Autodesk Inventor part; units mm, degrees
ref_plane "YZ Plane" through (0, 0, 0) normal (1, 0, 0) x (0, 1, 0)
ref_plane "XZ Plane" through (0, 0, 0) normal (0, 1, 0) x (-1, 0, 0)
ref_plane "XY Plane" through (0, 0, 0) normal (0, 0, 1) x (1, 0, 0)
sketch "Sketch1" plane through (0, 0, 0) normal (0, 0, 1) x (1, 0, 0)
  line L0 (-63.5, -76.2) -> (63.5, -76.2)
  line L1 (63.5, -76.2) -> (63.5, 76.2)
  line L2 (63.5, 76.2) -> (-63.5, 76.2)
  line L3 (-63.5, 76.2) -> (-63.5, -76.2)
  line L4 (-63.5, -76.2) -> (63.5, 76.2) construction
  line L5 (63.5, -76.2) -> (-63.5, 76.2) construction
  line L6 (-63.5, 76.2) -> (-50.0296, 62.7296)
  line L7 (-63.5, 76.2) -> (-44.45, 76.2) construction
  line L8 (63.5, 76.2) -> (69.85, 76.2) construction
  line L9 (63.5, 76.2) -> (50.0296, 62.7296)
  line L10 (63.5, -76.2) -> (50.0296, -62.7296)
  line L11 (-63.5, -76.2) -> (-50.0296, -62.7296)
  circle A0 centre (-50.0296, 62.7296) radius 3.175
  circle A1 centre (50.0296, 62.7296) radius 3.175
  circle A2 centre (50.0296, -62.7296) radius 3.175
  circle A3 centre (-50.0296, -62.7296) radius 3.175
  circle A4 centre (0, 0) radius 12.7
  line L12 (0, 0) -> (-48.4, 0) construction
  line L13 (0, 0) -> (12.7, 0)
  line L14 (0, 0) -> (49, 0) construction
  line L15 (49, 0) -> (49, 28.29) construction
  line L16 (49, 0) -> (49, -28.29) construction
  circle A5 centre (49, -28.29) radius 2.4
  circle A6 centre (49, 28.29) radius 2.4
  circle A7 centre (-48.4, 0) radius 2.4
  dimension "d10" = 25.4
  dimension "d0" = 127
  dimension "d1" = 152.4
  dimension "d2" = 19.05
  dimension "d3" = 45
  dimension "d6" = 6.35
  dimension "d7" = 6.35
  dimension "d8" = 6.35
  dimension "d9" = 6.35
  dimension "d11" = 48.4
  dimension "d12" = 49
  dimension "d13" = 28.29
  dimension "d14" = 28.29
  dimension "d15" = 4.8
  dimension "d16" = 4.8
  dimension "d17" = 4.8
extrude "Extrusion1" add sketch "Sketch1" along normal blind 6.35
properties part number "small plate"
Geometry check sheet. Reference: the model listing, model coordinates, mm. Coordinates: 2 decimals unless noted, no trailing zeros. Loops run counter-clockwise (first coordinate to the right, second up) from the corner with the lowest first, then second, coordinate; pieces in that order, holes last. Notation, with made-up numbers: (68.25, -8) - (109.25, -8) arc R29 ccw to (109.25, 23) - close; hole circle Ø11 at (80, 11.25). An arc over 180 degrees is marked (long way). One line per item, written item: value. Start each with the question number.
(1) Mould release check, pull along Y, two halves, no side actions. Record for faces 1 (the cylindrical face through (-50.798, -0.106, 3.131)), 2 (the flat face through (-63.5, 1, 3)), 3 (the flat face through (1, 76.2, 3)): released by +Y, released by -Y, zero draft, split by the parting line, or undercut.
(2) Depth check by flat-ended pin: P1, Ø8.5, axis at x = 50.03, y = 62.73, coming from the +Z side; P2, Ø23, axis at x = 0, y = 0, coming from the -Z side. Enter the tip coordinate at first touch or a pass-through.
(3) Cross-section at B-B on x = 0. Enter the section's corners in (y, z), plus the area to 3 significant figures.
(4) Material ranges on line 1 (X direction, y = -60, z = 5); line 2 (Y direction, x = 52.5, z = 2.25); line 3 (Y direction, x = 49, z = 4.5), recorded low to high. Write a range as [from, to].
(5) Cross-section at A-A on y = -28.29. Enter the section's corners in (x, z), plus the area to 3 significant figures.
(6) Cross-section at D-D on x = 49. Enter the section's corners in (y, z).
(7) Cross-section at C-C on z = 3. Count the separate pieces of the cut face and the enclosed holes in it, plus the area to 3 significant figures.
Results below:
1. face 1: undercut
1. face 2: zero draft
1. face 3: released by +Y
2. P1: stops at z = 6.35
2. P2: passes through
3. outline: (-76.2, 0) - (-12.7, 0) - (-12.7, 6.35) - (-76.2, 6.35) - close; (12.7, 0) - (76.2, 0) - (76.2, 6.35) - (12.7, 6.35) - close
3. area: 806 mm2
4. line 1: x = [-63.5, -51.65], [-48.41, 48.41], [51.65, 63.5]
4. line 2: y = [-76.2, -64.72], [-60.74, 60.74], [64.72, 76.2]
4. line 3: y = [-76.2, -65.73], [-59.73, -30.69], [-25.89, 25.89], [30.69, 59.73], [65.73, 76.2]
5. outline: (-63.5, 0) - (46.6, 0) - (46.6, 6.35) - (-63.5, 6.35) - close; (51.4, 0) - (63.5, 0) - (63.5, 6.35) - (51.4, 6.35) - close
5. area: 776 mm2
6. outline: (-76.2, 0) - (-65.73, 0) - (-65.73, 6.35) - (-76.2, 6.35) - close; (-59.73, 0) - (-30.69, 0) - (-30.69, 6.35) - (-59.73, 6.35) - close; (-25.89, 0) - (25.89, 0) - (25.89, 6.35) - (-25.89, 6.35) - close; (30.69, 0) - (59.73, 0) - (59.73, 6.35) - (30.69, 6.35) - close; (65.73, 0) - (76.2, 0) - (76.2, 6.35) - (65.73, 6.35) - close
7. separate pieces: 1
7. enclosed holes: 8
7. area: 18,700 mm2
